from build123d import *

# Parameters (mm, degrees)
SKETCH1_R           = 1.4
SKETCH1_W           = 20
SKETCH1_H           = 2
BOSS_EXTRUDE1_DEPTH = 7
SKETCH2_W           = 22
SKETCH2_H           = 4
SKETCH2_W_2         = 20
SKETCH2_H_2         = 2
CUT_EXTRUDE1_DEPTH  = 8.5
SKETCH3_R           = 39.79885979
CUT_EXTRUDE2_DEPTH  = 3


with BuildPart() as part:
    # Sketch1 → Boss-Extrude1 (new body)
    with BuildSketch(Plane.XY):
        with BuildLine():
            Line((-3, 0), (-3, -8))
            ThreePointArc((-3, -8), (-2.121320344, -10.121320344), (0, -11))
            Line((0, -11), (26, -11))
            ThreePointArc((26, -11), (28.121320344, -10.121320344), (29, -8))
            Line((29, -8), (29, 0))
            ThreePointArc((29, 0), (28.121320344, 2.121320344), (26, 3))
            Line((26, 3), (0, 3))
            ThreePointArc((0, 3), (-2.121320344, 2.121320344), (-3, 0))
        make_face()
        Circle(SKETCH1_R, mode=Mode.SUBTRACT)
        with Locations((0, -8)):
            Circle(SKETCH1_R, mode=Mode.SUBTRACT)
        with Locations((26, 0)):
            Circle(SKETCH1_R, mode=Mode.SUBTRACT)
        with Locations((26, -8)):
            Circle(SKETCH1_R, mode=Mode.SUBTRACT)
        with Locations((13, -4)):
            Rectangle(SKETCH1_W, SKETCH1_H, mode=Mode.SUBTRACT)
    extrude(amount=BOSS_EXTRUDE1_DEPTH)

    # Sketch2 → Cut-Extrude1 (cut)
    with BuildSketch(Plane.XY.offset(7)):
        with BuildLine():
            Line((26, 3), (0, 3))
            ThreePointArc((0, 3), (-2.121320344, 2.121320344), (-3, 0))
            Line((-3, 0), (-3, -8))
            ThreePointArc((-3, -8), (-2.121320344, -10.121320344), (0, -11))
            Line((0, -11), (26, -11))
            ThreePointArc((26, -11), (28.121320344, -10.121320344), (29, -8))
            Line((29, -8), (29, 0))
            ThreePointArc((29, 0), (28.121320344, 2.121320344), (26, 3))
        make_face()
        with BuildLine():
            Line((-2, -8), (-2, 0))
            ThreePointArc((-2, 0), (-1.414213562, 1.414213562), (0, 2))
            Line((0, 2), (26, 2))
            ThreePointArc((26, 2), (27.414213562, 1.414213562), (28, 0))
            Line((28, 0), (28, -8))
            ThreePointArc((28, -8), (27.414213562, -9.414213562), (26, -10))
            Line((26, -10), (0, -10))
            ThreePointArc((0, -10), (-1.414213562, -9.414213562), (-2, -8))
        make_face(mode=Mode.SUBTRACT)
        with Locations((13, -4)):
            Rectangle(SKETCH2_W, SKETCH2_H)
        with Locations((13, -4)):
            Rectangle(SKETCH2_W_2, SKETCH2_H_2, mode=Mode.SUBTRACT)
    extrude(amount=-CUT_EXTRUDE1_DEPTH, mode=Mode.SUBTRACT)

    # Sketch3 → Cut-Extrude2 (cut)
    with BuildSketch(Plane.XY.offset(7)):
        with Locations((0, 0.278776736)):
            Circle(SKETCH3_R)
    extrude(amount=-CUT_EXTRUDE2_DEPTH, mode=Mode.SUBTRACT)


solid = part.part
Source: CAD feature listing. Evaluate the final solid. Frame: model axes, mm. A direction names the side the tool comes from. Coordinates: 2 decimals unless noted, no trailing zeros. Loops run counter-clockwise (first coordinate to the right, second up) from the corner with the lowest first, then second, coordinate; pieces in that order, holes last. Notation, with made-up numbers: (58, -9) - (85, -9) arc R24 cw to (85, 14) - close; hole circle Ø3 at (80.25, -35.5). An arc over 180 degrees is marked (long way). One line per question, with ' | ' between items.
1) Pull-direction query (X, two-part tool) for faces 3 (the face through (-1.43, 1.4, 2.03)), 4 (the face through (13, -10, 2)), 5 (the face through (27.4, 1.43, 2.03)), 6 (the face through (27.29, -8.54, 1.97)); classes: released by +X, released by -X, zero draft, split by the parting line, or undercut.
Report:
face 3: released by -X | face 4: zero draft | face 5: released by +X | face 6: undercut
2) Section B-B, the plane x = 18. Return loops of the section in (y, z), then the cut area to 3 significant figures.
Report:
outline: (-10, 0) - (-6, 0) - (-6, 4) - (-10, 4) - close; (-2, 0) - (2, 0) - (2, 4) - (-2, 4) - close | area: 32.0 mm²
3) Line query: line 1 along Y through (x, z) = (0, 1.6); line 2 along X through (y, z) = (-8, 2.9); line 3 along Y through (x, z) = (23.25, 3.05). Output: solid intervals per line, ascending.
Report:
line 1: y = -10 to -9.4, -6.6 to -1.4, 1.4 to 2 | line 2: x = -2 to -1.4, 1.4 to 24.6, 27.4 to 28 | line 3: y = -10 to -6, -2 to 2
4) Section A-A, the plane y = -1. Return loops of the section in (x, z).
Report:
outline: (-2, 0) - (-0.98, 0) - (-0.98, 4) - (-2, 4) - close; (0.98, 0) - (25.02, 0) - (25.02, 4) - (0.98, 4) - close; (26.98, 0) - (28, 0) - (28, 4) - (26.98, 4) - close
5) Section C-C, the plane z = 1.35. Return loops of the section in (x, y), then the cut area to 3 significant figures.
Report:
outline: (-2, -8) arc R2 ccw to (0, -10) - (26, -10) arc R2 ccw to (28, -8) - (28, 0) arc R2 ccw to (26, 2) - (0, 2) arc R2 ccw to (-2, 0) - close; hole circle Ø2.8 at (0, -8); hole circle Ø2.8 at (0, 0); hole (2, -6) - (24, -6) - (24, -2) - (2, -2) - close; hole circle Ø2.8 at (26, -8); hole circle Ø2.8 at (26, 0) | area: 244 mm²
6) Set-up query: faces 1 (the face through (28, -4, 2)), 2 (the face through (2, -4, 2)). Return all of +Z, -Z, +X, -X, +Y, -Y with unobstructed straight access to the full face (end or side cutting, diameter ignored); none if empty.
Report:
face 1: +Z, -Z, +X, +Y, -Y | face 2: +Z, -Z
7) Section D-D, the plane y = -2.75. Return loops of the section in (x, z).
Report:
outline: (-2, 0) - (2, 0) - (2, 4) - (-2, 4) - close; (24, 0) - (28, 0) - (28, 4) - (24, 4) - close
